```python
from build123d import *

# Parameters (mm, degrees)
EXTRUDE_THIN1_DEPTH       = 12.7
F_6_CLEARANCE_HOLE1_D     = 3.7973
F_6_CLEARANCE_HOLE1_DEPTH = 7.62
F_6_CLEARANCE_HOLE1_TIP   = 1.140824014
F_6_CLEARANCE_HOLE2_D     = 3.7973
F_6_CLEARANCE_HOLE2_DEPTH = 7.62
F_6_CLEARANCE_HOLE2_TIP   = 1.140824014


with BuildPart() as part:
    # Sketch1 → Extrude-Thin1 (new body)
    with BuildSketch(Plane(origin=(0, 0, 0), x_dir=(0, 0, -1), z_dir=(1, 0, 0))):
        Polygon((-1.27, 15.748), (-1.27, 8.128), (60.325, 8.128), (60.325, 15.748), (62.865, 15.748), (62.865, 5.588), (-3.81, 5.588), (-3.81, 15.748), align=None)
    extrude(amount=EXTRUDE_THIN1_DEPTH)

    # #6 Clearance Hole1
    with Locations(Plane(origin=(0, 0, 1.27), x_dir=(-1, 0, 0), z_dir=(0, 0, -1))):
        with Locations((-6.35, 11.938)):
            Hole(F_6_CLEARANCE_HOLE1_D / 2, depth=F_6_CLEARANCE_HOLE1_DEPTH)
            with Locations((0, 0, -(F_6_CLEARANCE_HOLE1_DEPTH + F_6_CLEARANCE_HOLE1_TIP / 2))):  # 118° drill point
                Cone(0, F_6_CLEARANCE_HOLE1_D / 2, F_6_CLEARANCE_HOLE1_TIP, mode=Mode.SUBTRACT)

    # #6 Clearance Hole2
    with Locations(Plane.XY.offset(-60.325)):
        with Locations((6.35, 11.938)):
            Hole(F_6_CLEARANCE_HOLE2_D / 2, depth=F_6_CLEARANCE_HOLE2_DEPTH)
            with Locations((0, 0, -(F_6_CLEARANCE_HOLE2_DEPTH + F_6_CLEARANCE_HOLE2_TIP / 2))):  # 118° drill point
                Cone(0, F_6_CLEARANCE_HOLE2_D / 2, F_6_CLEARANCE_HOLE2_TIP, mode=Mode.SUBTRACT)


solid = part.part
```
Input: part model. Units: mm. Frame: model coordinates. A direction names the side the tool comes from. Give positions to 0.01 mm unless a question says otherwise; leave off trailing zeros. Order: outer loops, then holes, each group sorted by start corner. A loop starts at its lowest first (then second) coordinate and runs counter-clockwise, first axis right, second up.
1. Material intervals for L1, parallel to Z at x = 1.5, y = 11.5 (3 decimals); L2, parallel to Y at x = 6.35, z = -62; L3, parallel to Y at x = 4.5, z = -45, sorted ascending.
Derived:
L1: z = -62.865 to -60.325, 1.27 to 3.81
L2: y = 5.59 to 10.04, 13.84 to 15.75
L3: y = 5.59 to 8.13
2. Section B-B on x = 3. Return the cut outline in (y, z) (3 decimals).
Derived:
outline: (5.588, -62.865) - (15.748, -62.865) - (15.748, -60.325) - (8.128, -60.325) - (8.128, 1.27) - (15.748, 1.27) - (15.748, 3.81) - (5.588, 3.81) - close
3. Mould query, pull axis Y, two halves, no side actions, for faces 3 (the flat face through (6, 9, 3.81)), 4 (the cylindrical face through (6.6, 13.82, -61.61)), 5 (the flat face through (6, 15.748, -62)). Classes: released by +Y, released by -Y, zero draft, split by the parting line, or undercut.
Derived:
face 3: zero draft
face 4: undercut
face 5: released by +Y
4. Reachability of faces 1 (the flat face through (8, 14, -60.325)), 2 (the flat face through (0, 7, -30)) from +Z, -Z, +X, -X, +Y, -Y: full face, straight path, thin tool, end or side. Return the list, or none.
Derived:
face 1: +X, -X, +Y
face 2: +Z, -Z, -X, +Y, -Y
5. Pin query (flat end, axial travel): pin 1 (6.5 mm diameter, centred on x = 3.5, z = -17, fed in from +Y). Return the tip coordinate at first contact, or that it passes through.
Derived:
pin 1: stops at y = 8.13
6. Section C-C on z = -40. Return the cut outline in (x, y).
Derived:
outline: (0, 5.59) - (12.7, 5.59) - (12.7, 8.13) - (0, 8.13) - close
7. Section A-A on x = 6.35. Return the cut outline in (y, z) (3 decimals).
Derived:
outline: (5.588, -62.865) - (10.039, -62.865) - (10.039, -60.325) - (8.128, -60.325) - (8.128, 1.27) - (10.039, 1.27) - (10.039, 3.81) - (5.588, 3.81) - close; (13.837, -62.865) - (15.748, -62.865) - (15.748, -60.325) - (13.837, -60.325) - close; (13.837, 1.27) - (15.748, 1.27) - (15.748, 3.81) - (13.837, 3.81) - close
